```python
from build123d import *
from build123d.topology import SkipClean

# Parameters (mm, degrees)
SKETCH1_W                = 10
SKETCH1_H                = 80
SKETCH1_R                = 2.45
BOSS_EXTRUDE1_DEPTH      = 10
SKETCH2_W                = 10
SKETCH2_H                = 80
BOSS_EXTRUDE2_DEPTH      = 150
CUT_EXTRUDE1_DEPTH       = 166.227116419
SKETCH4_R                = 1.5
CUT_EXTRUDE2_DEPTH       = 301.861524459
SKETCH7_R                = 3.15
CUT_EXTRUDE5_DEPTH       = 10
SKETCH11_R               = 8.15
CUT_EXTRUDE7_DEPTH       = 5.2
SKETCH13_R               = 1.45
CUT_EXTRUDE8_DEPTH       = 5
CUT_EXTRUDE9_DEPTH       = 5
CUT_EXTRUDE10_DEPTH      = 5
CUT_EXTRUDE11_START      = -10
SKETCH16_R               = 2.4
CUT_EXTRUDE11_DEPTH      = 5
SKETCH17_R               = 1.5
BOSS_EXTRUDE4_DEPTH      = 6
SKETCH18_R               = 8.2
CUT_EXTRUDE12_DEPTH      = 6
SKETCH19_R               = 3
CUT_EXTRUDE13_DEPTH      = 10
SKETCH20_W               = 359.593382494
SKETCH20_H               = 674.632515804
CUT_EXTRUDE14_DEPTH      = 212.128383277
SKETCH22_R               = 1.45
CUT_EXTRUDE16_DEPTH      = 5
CUT_EXTRUDE17_DEPTH      = 166.290653093
CUT_EXTRUDE17_DEPTH_BACK = 166.290653093
CUT_EXTRUDE18_DEPTH      = 166.698521418
CUT_EXTRUDE18_DEPTH_BACK = 166.698521418
SKETCH24_W               = 8
SKETCH24_H               = 6


with BuildPart() as part:
    # Sketch1 → Boss-Extrude1 (new body)
    with BuildSketch(Plane(origin=(0, 0, 0), x_dir=(1, 0, 0), z_dir=(0, 1, 0))):
        with Locations((-120.815, 0)):
            Rectangle(SKETCH1_W, SKETCH1_H)
        with Locations(Location((-120.815, -31.75, 0), (0, 0, 270))):
            Circle(SKETCH1_R, mode=Mode.SUBTRACT)
        with Locations(Location((-120.815, -19.05, 0), (0, 0, 270))):
            Circle(SKETCH1_R, mode=Mode.SUBTRACT)
        with Locations(Location((-120.815, -6.35, 0), (0, 0, 270))):
            Circle(SKETCH1_R, mode=Mode.SUBTRACT)
        with Locations(Location((-120.815, 6.35, 0), (0, 0, 270))):
            Circle(SKETCH1_R, mode=Mode.SUBTRACT)
        with Locations(Location((-120.815, 19.05, 0), (0, 0, 270))):
            Circle(SKETCH1_R, mode=Mode.SUBTRACT)
        with Locations(Location((-120.815, 31.75, 0), (0, 0, 270))):
            Circle(SKETCH1_R, mode=Mode.SUBTRACT)
    extrude(amount=BOSS_EXTRUDE1_DEPTH)

    # Sketch2 → Boss-Extrude2 (add)
    with BuildSketch(Plane(origin=(0, 10, 0), x_dir=(1, 0, 0), z_dir=(0, 1, 0))):
        with Locations((-120.815, 0)):
            Rectangle(SKETCH2_W, SKETCH2_H)
    extrude(amount=BOSS_EXTRUDE2_DEPTH)

    # Sketch3 → Cut-Extrude1 (cut, through all)
    with BuildSketch(Plane.ZY.offset(125.815)):
        with BuildLine():
            Line((-40, 120), (-60, 120))
            Line((-60, 120), (-60, 170))
            Line((-60, 170), (60, 170))
            Line((60, 170), (60, 120))
            Line((60, 120), (40, 120))
            ThreePointArc((40, 120), (0, 160), (-40, 120))
        make_face()
    extrude(amount=-CUT_EXTRUDE1_DEPTH, mode=Mode.SUBTRACT)


with BuildPart() as body_2:
    # Mirror1: mirrored copy
    add(part.part.mirror(Plane(origin=(0, 0, 0), x_dir=(0, 0, 1), z_dir=(1, 0, 0))))


with BuildPart() as cut_extrude2_tool:
    # Sketch4 → Cut-Extrude2 (new, through all)
    with BuildSketch(Plane.ZY.offset(125.815)):
        with Locations((0, 120)):
            Circle(SKETCH4_R)
    extrude(amount=-CUT_EXTRUDE2_DEPTH)


with BuildPart() as part_1:
    add(part.part)

    # Cut-Extrude2: cut by cut_extrude2_tool
    add(cut_extrude2_tool.part, mode=Mode.SUBTRACT)

    # Sketch7 → Cut-Extrude5 (cut)
    with BuildSketch(Plane.ZY.offset(125.815)):
        with Locations((0, 120)):
            Circle(SKETCH7_R)
    extrude(amount=-CUT_EXTRUDE5_DEPTH, mode=Mode.SUBTRACT)

    # Sketch11 → Cut-Extrude7 (cut)
    with BuildSketch(Plane.ZY.offset(125.815)):
        with Locations((0, 120)):
            Circle(SKETCH11_R)
    extrude(amount=-CUT_EXTRUDE7_DEPTH, mode=Mode.SUBTRACT)

    # Sketch13 → Cut-Extrude8 (cut)
    with BuildSketch(Plane.ZY.offset(125.815)):
        with Locations((-12.5, 132.5)):
            Circle(SKETCH13_R)
        with Locations((12.5, 132.5)):
            Circle(SKETCH13_R)
        with Locations((12.5, 107.5)):
            Circle(SKETCH13_R)
        with Locations((-12.5, 107.5)):
            Circle(SKETCH13_R)
    extrude(amount=-CUT_EXTRUDE8_DEPTH, mode=Mode.SUBTRACT)

    # Sketch20 → Cut-Extrude14 (cut, through all)
    with BuildSketch(Plane(origin=(0, 0, 0), x_dir=(0, 0, -1), z_dir=(1, 0, 0))):
        Rectangle(SKETCH20_W, SKETCH20_H)
    extrude(amount=-CUT_EXTRUDE14_DEPTH, mode=Mode.SUBTRACT)


with BuildPart() as body_2_1:
    add(body_2.part)

    # Cut-Extrude2: cut by cut_extrude2_tool
    add(cut_extrude2_tool.part, mode=Mode.SUBTRACT)

    # Sketch14 → Cut-Extrude9 (cut)
    with BuildSketch(Plane(origin=(125.815, 0, 0), x_dir=(0, 0, -1), z_dir=(1, 0, 0))):
        with BuildLine():
            Line((25.4, 52.35), (13.104540125, 52.35))
            Line((13.104540125, 52.35), (10.650485711, 54.724046033))
            ThreePointArc((10.650485711, 54.724046033), (9.859214258, 55.56214504), (8.748782119, 55.871112549))
            Line((8.748782119, 55.871112549), (-8.748782119, 55.871112549))
            ThreePointArc((-8.748782119, 55.871112549), (-9.859214258, 55.56214504), (-10.650485712, 54.724046033))
            Line((-10.650485712, 54.724046033), (-13.104540125, 52.35))
            Line((-13.104540125, 52.35), (-25.4, 52.35))
            ThreePointArc((-25.4, 52.35), (-30.597234842, 50.197234842), (-32.75, 45))
            Line((-32.75, 45), (-32.75, 19.6))
            ThreePointArc((-32.75, 19.6), (-30.597234842, 14.402765158), (-25.4, 12.25))
            Line((-25.4, 12.25), (25.4, 12.25))
            ThreePointArc((25.4, 12.25), (30.597234842, 14.402765158), (32.75, 19.6))
            Line((32.75, 19.6), (32.75, 45))
            ThreePointArc((32.75, 45), (30.597234842, 50.197234842), (25.4, 52.35))
        make_face()
    extrude(amount=-CUT_EXTRUDE9_DEPTH, mode=Mode.SUBTRACT)

    # Sketch15 → Cut-Extrude10 (cut)
    with BuildSketch(Plane.ZY.offset(-115.815)):
        with BuildLine():
            Line((-9.899563657, 53.597002723), (-9.899563657, 16.29781068))
            ThreePointArc((-9.899563657, 16.29781068), (-9.533461074, 15.41396086), (-8.649611253, 15.047858277))
            Line((-8.649611253, 15.047858277), (8.649611253, 15.047858277))
            ThreePointArc((8.649611253, 15.047858277), (9.533461074, 15.41396086), (9.899563657, 16.29781068))
            Line((9.899563657, 16.29781068), (9.899563657, 53.597002723))
            ThreePointArc((9.899563657, 53.597002723), (9.607232135, 54.489704444), (8.748802207, 54.871112548))
            Line((8.748802207, 54.871112548), (-8.748802207, 54.871112548))
            ThreePointArc((-8.748802207, 54.871112548), (-9.607232135, 54.489704444), (-9.899563657, 53.597002723))
        make_face()
    extrude(amount=-CUT_EXTRUDE10_DEPTH, mode=Mode.SUBTRACT)

    # Sketch16 → Cut-Extrude11 (cut)
    with BuildSketch(Plane(origin=(125.815, 0, 0), x_dir=(0, 0, -1), z_dir=(1, 0, 0)).offset(CUT_EXTRUDE11_START)):
        with Locations((-25.4, 45)):
            Circle(SKETCH16_R)
        with Locations((-25.4, 32.3)):
            Circle(SKETCH16_R)
        with Locations((-25.4, 19.6)):
            Circle(SKETCH16_R)
        with Locations((25.4, 19.6)):
            Circle(SKETCH16_R)
        with Locations((25.4, 32.3)):
            Circle(SKETCH16_R)
        with Locations((25.4, 45)):
            Circle(SKETCH16_R)
    extrude(amount=CUT_EXTRUDE11_DEPTH, mode=Mode.SUBTRACT)

    # Sketch17 → Boss-Extrude4 (add)
    with SkipClean():  # the faces are left unmerged after this step: merging them gives an invalid solid
        with BuildSketch(Plane(origin=(125.815, 0, 0), x_dir=(0, 0, -1), z_dir=(1, 0, 0))):
            with BuildLine():
                ThreePointArc((40, 120), (0, 160), (-40, 120))
                Line((-40, 120), (-40, 0))
                Line((-40, 0), (40, 0))
                Line((40, 0), (40, 120))
            make_face()
            with BuildLine():
                Line((-13.104540125, 52.35), (-10.650485712, 54.724046033))
                ThreePointArc((-10.650485712, 54.724046033), (-9.859214258, 55.56214504), (-8.748782119, 55.871112549))
                Line((-8.748782119, 55.871112549), (8.748782119, 55.871112549))
                ThreePointArc((8.748782119, 55.871112549), (9.859214258, 55.56214504), (10.650485711, 54.724046033))
                Line((10.650485711, 54.724046033), (13.104540125, 52.35))
                Line((13.104540125, 52.35), (25.4, 52.35))
                ThreePointArc((25.4, 52.35), (30.597234842, 50.197234842), (32.75, 45))
                Line((32.75, 45), (32.75, 19.6))
                ThreePointArc((32.75, 19.6), (30.597234842, 14.402765158), (25.4, 12.25))
                Line((25.4, 12.25), (-25.4, 12.25))
                ThreePointArc((-25.4, 12.25), (-30.597234842, 14.402765158), (-32.75, 19.6))
                Line((-32.75, 19.6), (-32.75, 45))
                ThreePointArc((-32.75, 45), (-30.597234842, 50.197234842), (-25.4, 52.35))
                Line((-25.4, 52.35), (-13.104540125, 52.35))
            make_face(mode=Mode.SUBTRACT)
            with Locations((0, 120)):
                Circle(SKETCH17_R, mode=Mode.SUBTRACT)
        extrude(amount=BOSS_EXTRUDE4_DEPTH)

    # Sketch18 → Cut-Extrude12 (cut)
    with SkipClean():  # the faces are left unmerged after this step: merging them gives an invalid solid
        with BuildSketch(Plane(origin=(115.815, 0, 0), x_dir=(0, 0, -1), z_dir=(1, 0, 0))):
            with Locations((0, 120)):
                Circle(SKETCH18_R)
        extrude(amount=CUT_EXTRUDE12_DEPTH, mode=Mode.SUBTRACT)

    # Sketch19 → Cut-Extrude13 (cut)
    with BuildSketch(Plane.ZY.offset(-121.815)):
        with Locations((0, 120)):
            Circle(SKETCH19_R)
    extrude(amount=-CUT_EXTRUDE13_DEPTH, mode=Mode.SUBTRACT)

    # Sketch22 → Cut-Extrude16 (cut)
    with BuildSketch(Plane.ZY.offset(-115.815)):
        with Locations((-12.5, 107.5)):
            Circle(SKETCH22_R)
        with Locations((12.5, 107.5)):
            Circle(SKETCH22_R)
        with Locations((12.5, 132.5)):
            Circle(SKETCH22_R)
        with Locations((-12.5, 132.5)):
            Circle(SKETCH22_R)
    extrude(amount=-CUT_EXTRUDE16_DEPTH, mode=Mode.SUBTRACT)

    # Sketch23 → Cut-Extrude17 (cut, two sides: drawn at the far end of the back side and taken through both)
    with BuildSketch(Plane(origin=(120.815, 0, 0), x_dir=(0, 0, -1), z_dir=(1, 0, 0)).offset(-CUT_EXTRUDE17_DEPTH_BACK)):
        with BuildLine():
            Line((-8.649611253, 14.047858277), (8.649611253, 14.047858277))
            ThreePointArc((8.649611253, 14.047858277), (10.240567855, 14.706854078), (10.899563657, 16.29781068))
            Line((10.899563657, 16.29781068), (10.899563657, 53.554008783))
            ThreePointArc((10.899563657, 53.554008783), (10.329525513, 55.181625261), (8.748802207, 55.871112548))
            Line((8.748802207, 55.871112548), (-8.748802207, 55.871112548))
            ThreePointArc((-8.748802207, 55.871112548), (-10.329525513, 55.181625261), (-10.899563657, 53.554008783))
            Line((-10.899563657, 53.554008783), (-10.899563657, 16.29781068))
            ThreePointArc((-10.899563657, 16.29781068), (-10.240567855, 14.706854078), (-8.649611253, 14.047858277))
        make_face()
    extrude(amount=CUT_EXTRUDE17_DEPTH + CUT_EXTRUDE17_DEPTH_BACK, mode=Mode.SUBTRACT)

    # Sketch24 → Cut-Extrude18 (cut, two sides: drawn at the far end of the back side and taken through both)
    with BuildSketch(Plane(origin=(131.815, 0, 0), x_dir=(0, 0, -1), z_dir=(1, 0, 0)).offset(-CUT_EXTRUDE18_DEPTH_BACK)):
        with Locations((0, 58.871112549)):
            Rectangle(SKETCH24_W, SKETCH24_H)
    extrude(amount=CUT_EXTRUDE18_DEPTH + CUT_EXTRUDE18_DEPTH_BACK, mode=Mode.SUBTRACT)


solid = body_2_1.part
```
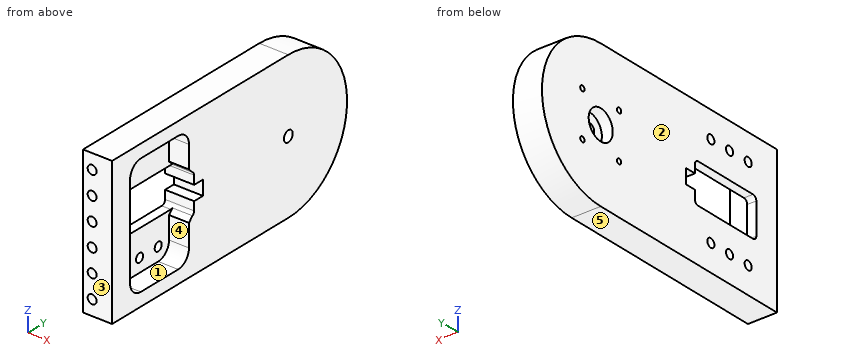
Source: CAD feature listing. Evaluate the final solid. Frame: model axes, mm. Face numbers are marked on the shaded views. A direction names the side the tool comes from. Round coordinates to 2 decimals unless told otherwise and drop trailing zeros. Loops run counter-clockwise (first coordinate to the right, second up) from the corner with the lowest first, then second, coordinate; pieces in that order, holes last. Notation, with made-up numbers: M -33.75,5 L -7.75,5 A16 ccw -7.75,19 Z; hole C 11.5,29.25 d11. An arc over 180 degrees is marked long. Use a Markdown table: item, result. Add a question column.
1. Cut plane C-C, the plane x = 128.5. State how many separate pieces and enclosed holes the cut face has, and give its area (3 significant figures).
2. Cut plane A-A, the plane y = 26. Output: boundary loops of the cut face in (x, z) (3 decimals), and give its area (3 significant figures).
3. Cut plane B-B, the plane z = 0. Output: boundary loops of the cut face in (x, y) (3 decimals), and give its area (3 significant figures).
4. Set-up query: the marked faces 1 and 2. Return all of +Z, -Z, +X, -X, +Y, -Y with unobstructed straight access to the full face (end or side cutting, diameter ignored); none if empty.
5. Ray query, line 1 along Y through (x, z) = (119.55, 0); line 2 along Z through (x, y) = (117.1, 107.5); line 3 along X through (y, z) = (7.5, 19.05) (3 decimals). Return the intervals inside material, ascending. Write a range as [from, to].
6. Contact query for flat-ended pins moving along their axis: pin 1 (5.5 mm diameter, centred on y = 19.6, z = 25.4, fed in from +X) (3 decimals); pin 2 (5 mm diameter, centred on x = 120, z = -25.5, fed in from +Y); pin 3 (9 mm diameter, centred on x = 128, z = -7, fed in from +Y). Output: stop coordinate, or through.
7. Cut plane D-D, the plane y = 132.5. Output: boundary loops of the cut face in (x, z) (3 decimals), and give its area (3 significant figures).
8. Pull-direction query (Y, two-part tool) for the marked faces 3, 4 and 5; classes: +Y half, -Y half, draft (parallel to the pull), parting line (faces both ways), or undercut.
Solution:
| question | item | result |
|---|---|---|
| 1 | separate pieces | 1 |
| 1 | enclosed holes | 2 |
| 1 | area | 9,380 mm2 |
| 2 | outline | M 115.815,-40 L 131.815,-40 L 131.815,-32.75 L 120.815,-32.75 L 120.815,-10.9 L 115.815,-10.9 Z; M 115.815,10.9 L 120.815,10.9 L 120.815,32.75 L 131.815,32.75 L 131.815,40 L 115.815,40 Z |
| 2 | area | 451 mm2 |
| 3 | outline | M 115.815,0 L 131.815,0 L 131.815,12.25 L 120.815,12.25 L 120.815,14.048 L 115.815,14.048 Z; M 115.815,61.871 L 131.815,61.871 L 131.815,117 L 121.815,117 L 121.815,111.8 L 115.815,111.8 Z; M 115.815,128.2 L 121.815,128.2 L 121.815,123 L 131.815,123 L 131.815,160 L 115.815,160 Z |
| 3 | area | 1,620 mm2 |
| 4 | face 1 | +X |
| 4 | face 2 | +Z, -Z, -X, +Y, -Y |
| 5 | line 1 | y = [0, 14.05], [61.87, 111.8], [128.2, 160] |
| 5 | line 2 | z = [-40, -13.95], [-11.05, 11.05], [13.95, 40] |
| 5 | line 3 | x = [115.815, 118.365], [123.265, 131.815] |
| 6 | pin 1 | stops at x = 120.815 |
| 6 | pin 2 | stops at y = 152.73 |
| 6 | pin 3 | stops at y = 159.92 |
| 7 | outline | M 115.815,-37.997 L 131.815,-37.997 L 131.815,37.997 L 115.815,37.997 L 115.815,13.95 L 120.815,13.95 L 120.815,11.05 L 115.815,11.05 L 115.815,-11.05 L 120.815,-11.05 L 120.815,-13.95 L 115.815,-13.95 Z |
| 7 | area | 1,190 mm2 |
| 8 | face 3 | -Y half |
| 8 | face 4 | undercut |
| 8 | face 5 | draft |
